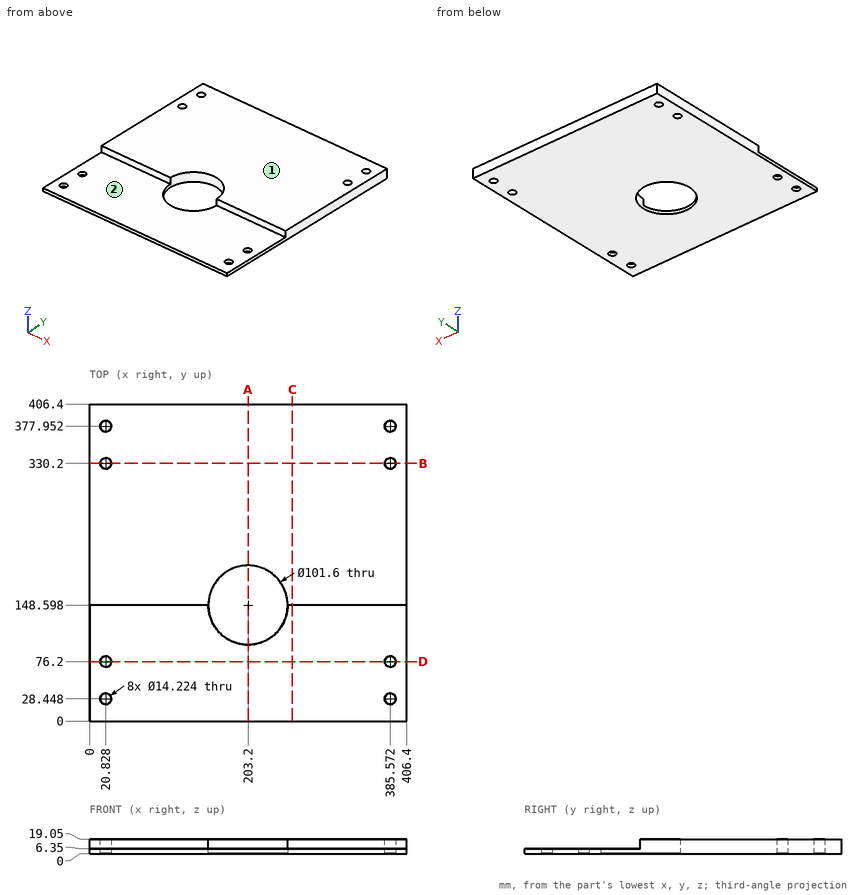
Geometry check sheet. Reference: drawing and pictorial views, mm from the part's lowest x, y, z. A direction names the side the tool comes from. Give positions to 0.01 mm unless a question says otherwise; leave off trailing zeros. Order: outer loops, then holes, each group sorted by start corner. A loop starts at its lowest first (then second) coordinate and runs counter-clockwise, first axis right, second up. Notation, with made-up numbers: M 88,82.25 L 127,82.25 A21 ccw 127,90.25 Z; hole C -21.75,89.25 d5. An arc over 180 degrees is marked long. Answer in a Markdown table with one row per item. Add a question column.
Item 1: Section check A-A, the plane x = 203.2. Enter the section's corners in (y, z), and give its area (3 significant figures).
Item 2: Section check B-B, the plane y = 330.2. Enter the section's corners in (x, z).
Item 3: Section check C-C, the plane x = 260. Enter the section's corners in (y, z).
Item 4: Scan lines: probe 1 along Y at (x, z) = (21.5, 1.75); probe 2 along X at (y, z) = (324, 11.25); probe 3 along X at (y, z) = (379.5, 6.5). Record each from-to range of solid material in increasing order. Write a range as from..to.
Item 5: Tool access check on the marked faces 1 and 2. Record the directions out of +Z, -Z, +X, -X, +Y, -Y that give a thin tool (end or side, any length) a straight path to the whole face; none if there is none.
Item 6: Gauge pin test, flat ends, axial feed: pin 1 (11.5 mm diameter, centred on x = 385.572, y = 377.952, fed in from -Z); pin 2 (6.5 mm diameter, centred on x = 328.5, z = 12, fed in from -Y); pin 3 (18.5 mm diameter, centred on x = 385.572, y = 76.2, fed in from +Z). Record the tip position at first contact, or that the pin passes through.
Item 7: Section check D-D, the plane y = 76.2. Enter the section's corners in (x, z), and give its area (3 significant figures).
Filled sheet:
| question | item | result |
|---|---|---|
| 1 | outline | M 0,0 L 97.8,0 L 97.8,6.35 L 0,6.35 Z; M 199.4,0 L 406.4,0 L 406.4,19.05 L 199.4,19.05 Z |
| 1 | area | 4,560 mm^2 |
| 2 | outline | M 0,0 L 13.72,0 L 13.72,19.05 L 0,19.05 Z; M 27.94,0 L 378.46,0 L 378.46,19.05 L 27.94,19.05 Z; M 392.68,0 L 406.4,0 L 406.4,19.05 L 392.68,19.05 Z |
| 3 | outline | M 0,0 L 406.4,0 L 406.4,19.05 L 148.6,19.05 L 148.6,6.35 L 0,6.35 Z |
| 4 | probe 1 | y = 0..21.37, 35.53..69.12, 83.28..323.12, 337.28..370.87, 385.03..406.4 |
| 4 | probe 2 | x = 0..17.34, 24.31..382.09, 389.06..406.4 |
| 4 | probe 3 | x = 0..13.89, 27.77..378.63, 392.51..406.4 |
| 5 | face 1 | +Z, +X, -X, +Y, -Y |
| 5 | face 2 | +Z, +X, -X, -Y |
| 6 | pin 1 | passes through |
| 6 | pin 2 | stops at y = 148.6 |
| 6 | pin 3 | stops at z = 6.35 |
| 7 | outline | M 0,0 L 13.72,0 L 13.72,6.35 L 0,6.35 Z; M 27.94,0 L 378.46,0 L 378.46,6.35 L 27.94,6.35 Z; M 392.68,0 L 406.4,0 L 406.4,6.35 L 392.68,6.35 Z |
| 7 | area | 2,400 mm^2 |
